```python
from build123d import *

# Parameters (mm, degrees)
CROQUIS2_R              = 1.5
SALIENTE_EXTRUIR1_DEPTH = 4
CROQUIS3_R              = 6
CROQUIS3_R_2            = 3.175
SALIENTE_EXTRUIR2_DEPTH = 12
CROQUIS4_R              = 1.5
CORTAR_EXTRUIR1_DEPTH   = 10


with BuildPart() as part:
    # Croquis2 → Saliente-Extruir1 (new body)
    with BuildSketch(Plane.XY):
        Polygon((3.608439182, 6.25), (-3.608439182, 6.25), (-7.216878365, 0), (-3.608439182, -6.25), (3.608439182, -6.25), (7.216878365, 0), align=None)
        Circle(CROQUIS2_R, mode=Mode.SUBTRACT)
    extrude(amount=SALIENTE_EXTRUIR1_DEPTH)

    # Croquis3 → Saliente-Extruir2 (add)
    with BuildSketch(Plane(origin=(0, 0, 0), x_dir=(-1, 0, 0), z_dir=(0, 0, -1))):
        Circle(CROQUIS3_R)
        Circle(CROQUIS3_R_2, mode=Mode.SUBTRACT)
    extrude(amount=SALIENTE_EXTRUIR2_DEPTH)

    # Croquis4 → Cortar-Extruir1 (cut)
    with BuildSketch(Plane(origin=(0, 0, 0), x_dir=(0, 0, -1), z_dir=(1, 0, 0))):
        with Locations((8.5, 0)):
            Circle(CROQUIS4_R)
    extrude(amount=CORTAR_EXTRUIR1_DEPTH, mode=Mode.SUBTRACT)


solid = part.part
```
Check sheet for the modelled part. Datum: model origin and axes. Units: mm. A direction names the side the tool comes from. Round coordinates to 2 decimals unless told otherwise and drop trailing zeros. Order: outer loops, then holes, each group sorted by start corner. A loop starts at its lowest first (then second) coordinate and runs counter-clockwise, first axis right, second up. Notation, with made-up numbers: (-33, 51) -> (-17, 51) arc R26 cw to (-17, 90) -> close; hole circle Ø4 at (-1, 14). An arc over 180 degrees is marked (long way). One line per item, written item: value. Start each with the question number.
Q1. Gauge pin test, flat ends, axial feed: pin 1 Ø2 at (x, z) = (5.5, 1.5) entering from -Y; pin 2 Ø2 at (y, z) = (3, -2) entering from +X; pin 3 Ø6 at (x, z) = (-3.5, -6) entering from -Y. Record the tip position at first contact, or that the pin passes through.
Q2. Mould release check, pull along X, two halves, no side actions. Record for faces 1 (the face through (-5.44, -3.08, 1.97)), 2 (the face through (-3, -3, -12)), 3 (the face through (0.7, 1.5, 0)): pulls with the +X half, pulls with the -X half, needs draft (parallel to the pull), parting line crosses it, or undercut.
Q3. Thickness scan on line 1 (Y direction, x = 0, z = 1.1); line 2 (X direction, y = 0, z = -4.5) (3 decimals). Record the ranges inside material, lowest first.
Q4. Cross-section at C-C (y = -0.75). Record the boundary of the cut face in (x, z).
Q5. Cross-section at A-A (z = 1). Record the boundary of the cut face in (x, y).
Q6. Cross-section at D-D (y = -3.75). Record the boundary of the cut face in (x, z).
Q7. Set-up check for faces 4 (the face through (0, 6.25, 2)), 5 (the face through (-5.723, 1.802, -5.916)), 6 (the face through (4.377, -0.575, -9.886)): record each of +Z, -Z, +X, -X, +Y, -Y from which the full face is reachable in a straight line by a thin tool's end or side.
Q8. Cross-section at B-B (x = 0). Record the boundary of the cut face in (y, z) (3 decimals).
Completed:
1. pin 1: stops at y = -4.71
1. pin 2: stops at x = 5.66
1. pin 3: stops at y = -5.98
2. face 1: pulls with the -X half
2. face 2: needs draft
2. face 3: undercut
3. line 1: y = -6.25 to -1.5, 1.5 to 6.25
3. line 2: x = -6 to -3.175, 3.175 to 6
4. outline: (-6.78, 0) -> (-5.95, 0) -> (-5.95, -12) -> (-3.09, -12) -> (-3.09, 0) -> (-1.3, 0) -> (-1.3, 4) -> (-6.78, 4) -> close; (1.3, 0) -> (3.09, 0) -> (3.09, -7.2) -> (5.95, -7.2) -> (5.95, 0) -> (6.78, 0) -> (6.78, 4) -> (1.3, 4) -> close; (3.09, -12) -> (5.95, -12) -> (5.95, -9.8) -> (3.09, -9.8) -> close
5. outline: (-7.22, 0) -> (-3.61, -6.25) -> (3.61, -6.25) -> (7.22, 0) -> (3.61, 6.25) -> (-3.61, 6.25) -> close; hole circle Ø3 at (0, 0)
6. outline: (-5.05, 0) -> (-4.68, 0) -> (-4.68, -12) -> (4.68, -12) -> (4.68, 0) -> (5.05, 0) -> (5.05, 4) -> (-5.05, 4) -> close
7. face 4: +Z, -Z, +X, -X, +Y
7. face 5: -Z
7. face 6: +X
8. outline: (-6.25, 0) -> (-6, 0) -> (-6, -12) -> (-3.175, -12) -> (-3.175, 0) -> (-1.5, 0) -> (-1.5, 4) -> (-6.25, 4) -> close; (1.5, 0) -> (3.175, 0) -> (3.175, -12) -> (6, -12) -> (6, 0) -> (6.25, 0) -> (6.25, 4) -> (1.5, 4) -> close
